The model under review builds one solid part; all positions refer to its coordinate system, in mm. Face numbers are marked on the shaded views. A direction names the side the tool comes from. Give positions to 0.01 mm unless a question says otherwise; leave off trailing zeros. Order: outer loops, then holes, each group sorted by start corner. A loop starts at its lowest first (then second) coordinate and runs counter-clockwise, first axis right, second up.
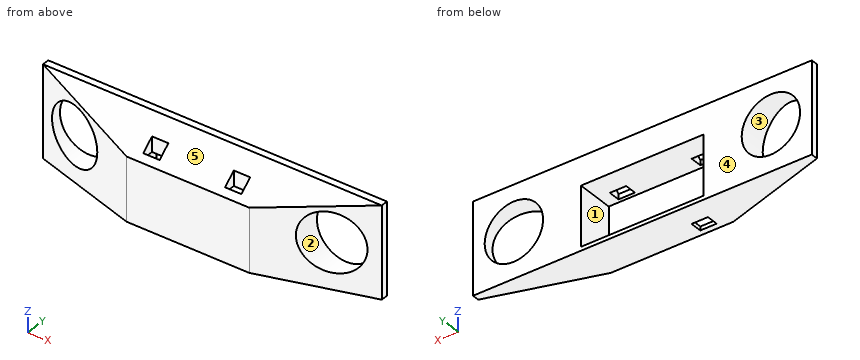
```python
from build123d import *

# Parameters (mm, degrees)
F0_W      = 145
F0_H      = 39
F0_R      = 12.5
F1_DEPTH  = 17
F4_DEPTH  = 300
F6_DEPTH  = 100
F7_W      = 7
F7_H      = 5
F8_DEPTH  = 200
F9_W      = 10.465479
F9_H      = 7.249243
F10_DEPTH = 3
F11_W     = 52.539315
F11_H     = 25.348472
F12_DEPTH = 16


with BuildPart() as f1:
    # F0 (on Front) → F1 (new body)
    with BuildSketch(Plane.XZ):
        Rectangle(F0_W, F0_H)
        with Locations((-55, 0)):
            Circle(F0_R, mode=Mode.SUBTRACT)
        with Locations((55, 0)):
            Circle(F0_R, mode=Mode.SUBTRACT)
    extrude(amount=F1_DEPTH)

    # F3 (on face) → F4 (cut)
    with BuildSketch(Plane(origin=(-72.5, 0, 0), x_dir=(0, -1, 0), z_dir=(-1, 0, 0))):
        Polygon((3, 19.5), (17, 7.5), (17, 19.5), align=None)
    extrude(amount=-F4_DEPTH, mode=Mode.SUBTRACT)

    # F5 (on face) → F6 (cut)
    with BuildSketch(Plane(origin=(0, 0, -19.5), x_dir=(1, 0, 0), z_dir=(0, 0, -1))):
        Polygon((-72.5, 3), (-26.25, 17), (-72.5, 17), align=None)
        Polygon((72.5, 17), (26.25, 17), (72.5, 3), align=None)
    extrude(amount=-F6_DEPTH, mode=Mode.SUBTRACT)

    # F7 (on face) → F8 (cut)
    with BuildSketch(Plane(origin=(0, 0, -19.5), x_dir=(1, 0, 0), z_dir=(0, 0, -1))):
        with Locations((-17.5, 12)):
            Rectangle(F7_W, F7_H)
        with Locations((17.5, 12)):
            Rectangle(F7_W, F7_H)
    extrude(amount=-F8_DEPTH, mode=Mode.SUBTRACT)

    # F9 (on face) → F10 (join)
    with BuildSketch(Plane(origin=(0, 0, -19.5), x_dir=(1, 0, 0), z_dir=(0, 0, -1))):
        with Locations((17.402842, 12.139229)):
            Rectangle(F9_W, F9_H)
    extrude(amount=-F10_DEPTH)

    # F11 (on face) → F12 (cut)
    with BuildSketch(Plane(origin=(0, 0, 0), x_dir=(-1, 0, 0), z_dir=(0, 1, 0))):
        with Locations((-0.041759, -5.197565)):
            Rectangle(F11_W, F11_H)
    extrude(amount=-F12_DEPTH, mode=Mode.SUBTRACT)


solid = f1.part
```
Item 1: Take a section at B-B (z = 5). Give the boundary of the cut face in (x, y).
Values found:
outline: (-72.5, -3) - (-66.46, -4.83) - (-66.46, 0) - (-72.5, 0) - close; (-43.54, -11.77) - (-26.25, -17) - (26.25, -17) - (43.54, -11.77) - (43.54, 0) - (26.31, 0) - (26.31, -16) - (-26.23, -16) - (-26.23, 0) - (-43.54, 0) - close; (66.46, -4.83) - (72.5, -3) - (72.5, 0) - (66.46, 0) - close
Item 2: For line 1 (X direction, y = -1.5, z = -0.5); line 2 (X direction, y = -7.5, z = 0); line 3 (Z direction, x = -55, y = -3), list the stretches that pass through material, from the lowest coordinate up.
Values found:
line 1: x = -72.5 to -67.49, -42.51 to -26.23, 26.31 to 42.51, 67.49 to 72.5
line 2: x = -42.5 to -26.23, 26.31 to 42.5
line 3: z = -19.5 to -12.5, 12.5 to 19.5
Item 3: Draft analysis for pull direction Z (two halves, no side actions). For the marked faces 3, 4 and 5, state which applies: released by +Z, released by -Z, zero draft, split by the parting line, or undercut.
Values found:
face 3: undercut
face 4: zero draft
face 5: released by +Z
Item 4: Clearance check with flat-ended pins moving along their axes: pin 1 Ø5.5 at (y, z) = (-11, 9.5) entering from +X; pin 2 Ø15 at (x, z) = (55, 0) entering from +Y; pin 3 Ø5 at (x, y) = (42.5, -14) entering from +Z; pin 4 Ø6 at (x, y) = (28, -6.5) entering from +Z. State where each tip first meets the part, or that it passes through.
Values found:
pin 1: stops at x = 50.94
pin 2: passes through
pin 3: stops at z = 12.21
pin 4: stops at z = 19.07
Item 5: For the marked faces 1 and 2, list the 3-axis set-ups (+Z, -Z, +X, -X, +Y, -Y) from which the entire face can be reached by the end or side of a thin tool; tool diameter is ignored.
Values found:
face 1: +Y
face 2: +Y, -Y
Item 6: Take a section at A-A (x = 53). Give the boundary of the cut face in (y, z), and give its area (3 significant figures).
Values found:
outline: (-8.9, -19.5) - (0, -19.5) - (0, -12.34) - (-8.9, -12.34) - close; (-8.9, 12.34) - (0, 12.34) - (0, 19.5) - (-3, 19.5) - (-8.9, 14.44) - close
area: 113 mm2
Item 7: Take a section at C-C (z = 15.5). Give the boundary of the cut face in (x, y).
Values found:
outline: (-72.5, -3) - (-57.08, -7.67) - (57.08, -7.67) - (72.5, -3) - (72.5, 0) - (-72.5, 0) - close
Item 8: Take a section at D-D (x = -35). Give the boundary of the cut face in (y, z).
Values found:
outline: (-14.35, -19.5) - (0, -19.5) - (0, 19.5) - (-3, 19.5) - (-14.35, 9.77) - close
